The model under review builds one solid part; all positions refer to its coordinate system, in mm. Face numbers are marked on the shaded views. A direction names the side the tool comes from. Give positions to 0.01 mm unless a question says otherwise; leave off trailing zeros. Write each loop counter-clockwise with the first axis right and the second up, starting at its lowest first coordinate (ties: lowest second). Pieces come first, ordered by that corner, then holes. Notation, with made-up numbers: M -35.5,36 L 22.5,36 A9 ccw 22.5,48 Z; hole C 19.5,-9.75 d10. An arc over 180 degrees is marked long. Write item = value, one per line. Start each with the question number.
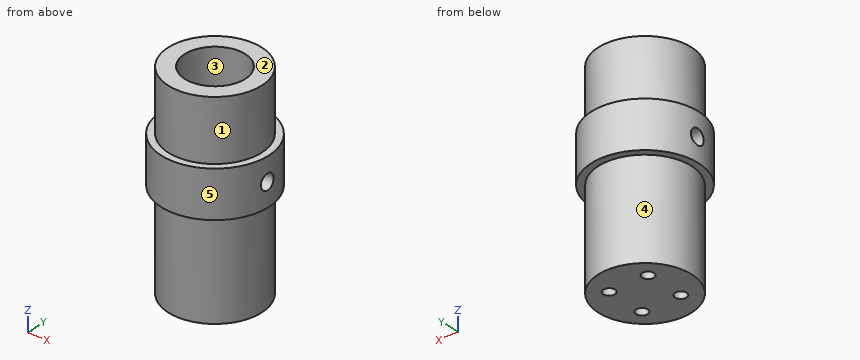
```python
from build123d import *

# Parameters (mm, degrees)
SKETCH_1_R          = 10
EXTRUDE_1_DEPTH     = 44
SKETCH_2_R          = 6.5
CUT_EXTRUDE_1_DEPTH = 27
M3X0_51_D           = 2.5
M3X0_51_DEPTH       = 8.5
M3X0_51_TIP         = 0.751075774
SKETCH_10_R         = 11.5
SKETCH_10_R_2       = 10
EXTRUDE_2_DEPTH     = 10
M4X0_71_D           = 3.3


with BuildPart() as part:
    # Эскиз1 → Бобышка-Вытянуть1 (new body)
    with BuildSketch(Plane.XY):
        Circle(SKETCH_1_R)
    extrude(amount=EXTRUDE_1_DEPTH)

    # Эскиз2 → Вырез-Вытянуть1 (cut)
    with BuildSketch(Plane.XY.offset(44)):
        Circle(SKETCH_2_R)
    extrude(amount=-CUT_EXTRUDE_1_DEPTH, mode=Mode.SUBTRACT)

    # Отверстие обработанное метчиком M3x0.51
    with Locations(Plane(origin=(0, 0, 0), x_dir=(-1, 0, 0), z_dir=(0, 0, -1))):
        with Locations((-4.242640687, 4.242640687), (4.242640687, 4.242640687), (4.242640687, -4.242640687), (-4.242640687, -4.242640687)):
            Hole(M3X0_51_D / 2, depth=M3X0_51_DEPTH)
            with Locations((0, 0, -(M3X0_51_DEPTH + M3X0_51_TIP / 2))):  # 118° drill point
                Cone(0, M3X0_51_D / 2, M3X0_51_TIP, mode=Mode.SUBTRACT)

    # Эскиз10 → Бобышка-Вытянуть2 (add)
    with BuildSketch(Plane(origin=(0, 0, 21), x_dir=(-1, 0, 0), z_dir=(0, 0, -1))):
        Circle(SKETCH_10_R)
        Circle(SKETCH_10_R_2, mode=Mode.SUBTRACT)
    extrude(amount=-EXTRUDE_2_DEPTH)

    # Отверстие обработанное метчиком M4x0.71 (through all)
    with Locations(Plane(origin=(-11.5, 0, 0), x_dir=(0, 0, -1), z_dir=(-1, 0, 0))):
        with Locations((-26, 0)):
            Hole(M4X0_71_D / 2)


solid = part.part
```
Item 1: Clearance check with flat-ended pins moving along their axes: P1, Ø2, axis at x = -4.24, y = -4.24, coming from the -Z side; P2, Ø5, axis at y = -3.5, z = 17.5, coming from the -X side; P3, Ø2, axis at y = 0.5, z = 34, coming from the -X side. State where each tip first meets the part, or that it passes through.
Item 2: We need section C-C, the plane x = 0. Write out the cut boundary in (y, z).
Item 3: We need section A-A, the plane y = 0. Write out the cut boundary in (x, z).
Item 4: We need section B-B, the plane z = 26. Write out the cut boundary in (x, y), and give its area (3 significant figures).
Item 5: To check wall thickness, follow probe 1 along X at (y, z) = (-4.25, 5); probe 2 along Z at (x, y) = (-2.25, 4); probe 3 along Z at (x, y) = (-3.25, -9.5). State the ranges of each line that lie inside material, in increasing order. Write a range as [from, to].
Item 6: For the marked faces 4 and 5, list the 3-axis set-ups (+Z, -Z, +X, -X, +Y, -Y) from which the entire face can be reached by the end or side of a thin tool; tool diameter is ignored.
Item 7: We need section D-D, the plane y = 7. Write out the cut boundary in (x, z).
Item 8: The part is to be moulded in two halves that separate along X. For the marked faces 1, 2 and 3, say which applies: released by +X, released by -X, zero draft, split by the parting line, or undercut.
Worked out:
q1.P1 = 8.65
q1.P2 = -9.95
q1.P3 = -10
q2.outline = M -11.5,21 L -10,21 L -10,0 L 10,0 L 10,21 L 11.5,21 L 11.5,31 L 10,31 L 10,44 L 6.5,44 L 6.5,17 L -6.5,17 L -6.5,44 L -10,44 L -10,31 L -11.5,31 Z
q3.outline = M -11.5,21 L -10,21 L -10,0 L 10,0 L 10,21 L 11.5,21 L 11.5,24.35 L 6.5,24.35 L 6.5,17 L -6.5,17 L -6.5,24.35 L -11.5,24.35 Z; M -11.5,27.65 L -6.5,27.65 L -6.5,44 L -10,44 L -10,31 L -11.5,31 Z; M 6.5,27.65 L 11.5,27.65 L 11.5,31 L 10,31 L 10,44 L 6.5,44 Z
q4.outline = M -11.38,-1.65 A11.5 ccw 11.38,-1.65 L 6.29,-1.65 A6.5 cw -6.29,-1.65 Z; M -11.38,1.65 L -6.29,1.65 A6.5 cw 6.29,1.65 L 11.38,1.65 A11.5 ccw Z
q4.area = 250 mm²
q5.probe_1 = [-9.05, -5.49], [-2.99, 2.99], [5.49, 9.05]
q5.probe_2 = [0, 17]
q5.probe_3 = [21, 31]
q6.face_4 = -Z
q6.face_5 = +Z, -Z
q7.outline = M -9.12,21 L -7.14,21 L -7.14,0 L 7.14,0 L 7.14,21 L 9.12,21 L 9.12,31 L 7.14,31 L 7.14,44 L -7.14,44 L -7.14,31 L -9.12,31 Z
q8.face_1 = split by the parting line
q8.face_2 = zero draft
q8.face_3 = undercut
